Check sheet for the modelled part. Datum: model origin and axes. Units: mm. Face numbers are marked on the shaded views. A direction names the side the tool comes from. Give positions to 0.01 mm unless a question says otherwise; leave off trailing zeros. Write each loop counter-clockwise with the first axis right and the second up, starting at its lowest first coordinate (ties: lowest second). Pieces come first, ordered by that corner, then holes. Notation, with made-up numbers: (89.5, 24.5) -> (95.5, 24.5) arc R18 ccw to (95.5, 47.5) -> close; hole circle Ø10 at (49, 78.5). An arc over 180 degrees is marked (long way). Return JSON: item names as keys, results as strings.
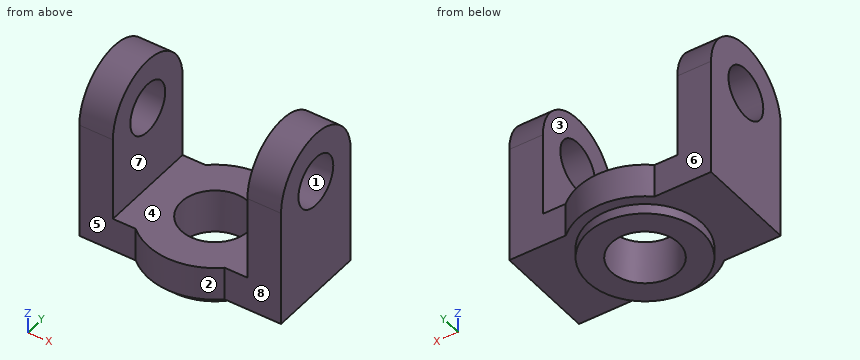
from build123d import *

# Parameters (mm, degrees)
F0_R     = 10
F1_DEPTH = 10
F2_R     = 17
F2_R_2   = 10
F3_DEPTH = 3
F4_R     = 7.5
F5_DEPTH = 10
F6_R     = 7.5
F7_DEPTH = 10


with BuildPart() as f1:
    # F0 (on Top) → F1 (new body)
    with BuildSketch(Plane.XY):
        with BuildLine():
            Line((6.7712434447, 0), (0, 0))
            Line((0, 0), (0, -15))
            ThreePointArc((0, -15), (1.7712434447, -6.7712434447), (6.7712434447, 0))
        make_face()
        with BuildLine():
            ThreePointArc((6.7712434447, -30), (1.7712434447, -23.2287565553), (0, -15))
            Line((0, -15), (0, -30))
            Line((0, -30), (6.7712434447, -30))
        make_face()
        with BuildLine():
            Line((40, 0), (33.2287565553, 0))
            ThreePointArc((33.2287565553, 0), (38.2287565553, -6.7712434447), (40, -15))
            Line((40, -15), (40, 0))
        make_face()
        with BuildLine():
            Line((40, -30), (40, -15))
            ThreePointArc((40, -15), (38.2287565553, -23.2287565553), (33.2287565553, -30))
            Line((33.2287565553, -30), (40, -30))
        make_face()
        with BuildLine():
            Line((33.2287565553, 0), (6.7712434447, 0))
            ThreePointArc((6.7712434447, 0), (1.7712434447, -6.7712434447), (0, -15))
            ThreePointArc((0, -15), (1.7712434447, -23.2287565553), (6.7712434447, -30))
            Line((6.7712434447, -30), (33.2287565553, -30))
            ThreePointArc((33.2287565553, -30), (38.2287565553, -23.2287565553), (40, -15))
            ThreePointArc((40, -15), (38.2287565553, -6.7712434447), (33.2287565553, 0))
        make_face()
        with Locations((20, -15)):
            Circle(F0_R, mode=Mode.SUBTRACT)
        with BuildLine():
            ThreePointArc((33.2287565553, 0), (20, 5), (6.7712434447, 0))
            Line((6.7712434447, 0), (33.2287565553, 0))
        make_face()
        with BuildLine():
            Line((33.2287565553, -30), (6.7712434447, -30))
            ThreePointArc((6.7712434447, -30), (20, -35), (33.2287565553, -30))
        make_face()
    extrude(amount=F1_DEPTH)

    # F2 (on face) → F3 (join)
    with BuildSketch(Plane(origin=(0, 0, 0), x_dir=(1, 0, 0), z_dir=(0, 0, -1))):
        with Locations((20, 15)):
            Circle(F2_R)
        with Locations((20, 15)):
            Circle(F2_R_2, mode=Mode.SUBTRACT)
    extrude(amount=F3_DEPTH)

    # F4 (on face) → F5 (join)
    with BuildSketch(Plane.YZ.offset(40)):
        with BuildLine():
            Line((-30, 35), (-30, 0))
            Line((-30, 0), (0, 0))
            Line((0, 0), (0, 35))
            ThreePointArc((0, 35), (-15, 50), (-30, 35))
        make_face()
        with Locations((-15, 35)):
            Circle(F4_R, mode=Mode.SUBTRACT)
    extrude(amount=F5_DEPTH)

    # F6 (on face) → F7 (join)
    with BuildSketch(Plane(origin=(0, 0, 0), x_dir=(0, -1, 0), z_dir=(-1, 0, 0))):
        with BuildLine():
            ThreePointArc((30, 35), (15, 50), (0, 35))
            Line((0, 35), (0, 0))
            Line((0, 0), (30, 0))
            Line((30, 0), (30, 35))
        make_face()
        with Locations((15, 35)):
            Circle(F6_R, mode=Mode.SUBTRACT)
    extrude(amount=F7_DEPTH)


solid = f1.part
(1) Cross-section at A-A on x = 20. Enter the section's corners in (y, z).
Reply:
{"outline": "(-35, 0) -> (-32, 0) -> (-32, -3) -> (-25, -3) -> (-25, 10) -> (-35, 10) -> close; (-5, -3) -> (2, -3) -> (2, 0) -> (5, 0) -> (5, 10) -> (-5, 10) -> close"}
(2) Cross-section at C-C on y = -15. Enter the section's corners in (x, z), then the cut area to 3 significant figures.
Reply:
{"outline": "(-10, 0) -> (3, 0) -> (3, -3) -> (10, -3) -> (10, 10) -> (0, 10) -> (0, 27.5) -> (-10, 27.5) -> close; (-10, 42.5) -> (0, 42.5) -> (0, 50) -> (-10, 50) -> close; (30, -3) -> (37, -3) -> (37, 0) -> (50, 0) -> (50, 27.5) -> (40, 27.5) -> (40, 10) -> (30, 10) -> close; (40, 42.5) -> (50, 42.5) -> (50, 50) -> (40, 50) -> close", "area": "942 mm^2"}
(3) Set-up check for the marked faces 5, 6, 7 and 8: record each of +Z, -Z, +X, -X, +Y, -Y from which the full face is reachable in a straight line by a thin tool's end or side.
Reply:
{"face 5": "+Z, -Z, -X, -Y", "face 6": "+Z, -Z, -X, +Y", "face 7": "+Z, +Y, -Y", "face 8": "+Z, -Z, +X, -Y"}
(4) Cross-section at D-D on y = -6.5. Enter the section's corners in (x, z).
Reply:
{"outline": "(-10, 0) -> (5.28, 0) -> (5.28, -3) -> (14.73, -3) -> (14.73, 10) -> (0, 10) -> (0, 47.36) -> (-10, 47.36) -> close; (25.27, -3) -> (34.72, -3) -> (34.72, 0) -> (50, 0) -> (50, 47.36) -> (40, 47.36) -> (40, 10) -> (25.27, 10) -> close"}
(5) Cross-section at B-B on z = 18.5. Enter the section's corners in (x, y).
Reply:
{"outline": "(-10, -30) -> (0, -30) -> (0, 0) -> (-10, 0) -> close; (40, -30) -> (50, -30) -> (50, 0) -> (40, 0) -> close"}
(6) Depth check by flat-ended pin: pin 1 Ø8.5 at (x, z) = (-0.5, 19.5) entering from -Y; pin 2 Ø18.5 at (x, z) = (-1.5, 21.5) entering from +Y; pin 3 Ø3 at (x, y) = (19.5, -2) entering from +Z. Enter the tip coordinate at first touch or a pass-through.
Reply:
{"pin 1": "y = -30", "pin 2": "y = 0", "pin 3": "z = 10"}
(7) Release check for a two-part mould opening along X. For the marked faces 1, 2, 3 and 4 record: pulls with the +X half, pulls with the -X half, needs draft (parallel to the pull), parting line crosses it, or undercut.
Reply:
{"face 1": "needs draft", "face 2": "parting line crosses it", "face 3": "undercut", "face 4": "undercut"}
(8) Thickness scan on L1, parallel to X at y = -11.5, z = 10.5; L2, parallel to Z at x = -3.75, y = -15; L3, parallel to X at y = -15, z = 0.75. Record the ranges inside material, lowest first.
Reply:
{"L1": "-10 to 0, 40 to 50", "L2": "0 to 27.5, 42.5 to 50", "L3": "-10 to 10, 30 to 50"}
